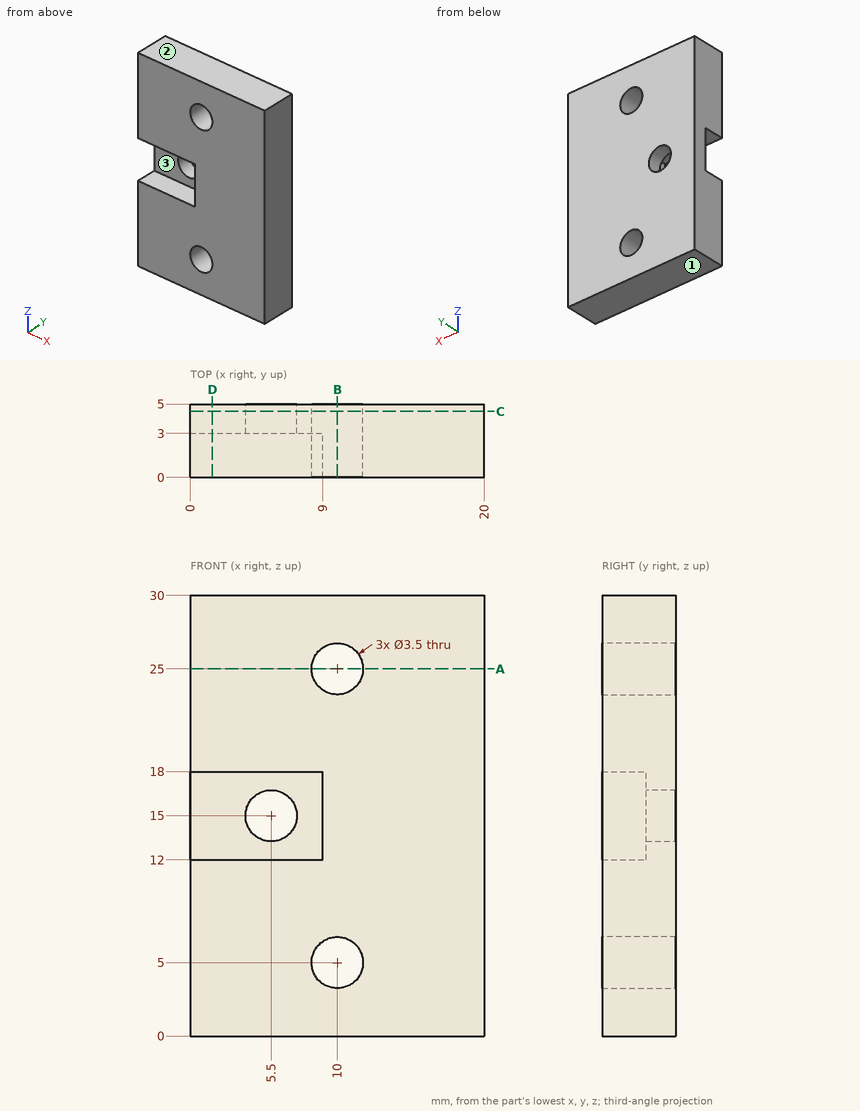
Design review of the part shown in the three views and the two pictorial views. Dimensions are in mm from the part's minimum x, y and z. Round coordinates to 2 decimals unless told otherwise and drop trailing zeros. Order: outer loops, then holes, each group sorted by start corner. A loop starts at its lowest first (then second) coordinate and runs counter-clockwise, first axis right, second up.
(1) Take a section at C-C, the plane y = 4.5. State the section outline as (x, z) points, plus the area to 3 significant figures.
Working result:
outline: (0, 0) - (20, 0) - (20, 30) - (0, 30) - close; hole circle Ø3.5 at (5.5, 15); hole circle Ø3.5 at (10, 5); hole circle Ø3.5 at (10, 25)
area: 571 mm2
(2) For P1, Ø3, axis at x = 6, z = 14.5, coming from the -Y side; P2, Ø0.9, axis at y = 1.5, z = 16.5, coming from the -X side, all flat-tipped, find the tip position at first contact; note any pin that passes through.
Working result:
P1: stops at y = 3
P2: stops at x = 9
(3) Wall thickness on L1, parallel to X at y = 3.9, z = 15; L2, parallel to X at y = 1.9, z = 25; L3, parallel to Z at x = 9.25, y = 1.35: over which ranges is each line inside the solid? List them lowest first.
Working result:
L1: x = 0 to 3.75, 7.25 to 20
L2: x = 0 to 8.25, 11.75 to 20
L3: z = 0 to 3.42, 6.58 to 23.42, 26.58 to 30
(4) Take a section at D-D, the plane x = 1.5. State the section outline as (y, z) points.
Working result:
outline: (0, 0) - (5, 0) - (5, 30) - (0, 30) - (0, 18) - (3, 18) - (3, 12) - (0, 12) - close
(5) Take a section at A-A, the plane z = 25. State the section outline as (x, y) points.
Working result:
outline: (0, 0) - (8.25, 0) - (8.25, 5) - (0, 5) - close; (11.75, 0) - (20, 0) - (20, 5) - (11.75, 5) - close
(6) Take a section at B-B, the plane x = 10. State the section outline as (y, z) points, plus the area to 3 significant figures.
Working result:
outline: (0, 0) - (5, 0) - (5, 3.25) - (0, 3.25) - close; (0, 6.75) - (5, 6.75) - (5, 23.25) - (0, 23.25) - close; (0, 26.75) - (5, 26.75) - (5, 30) - (0, 30) - close
area: 115 mm2
(7) Mouldability with a two-part tool opening along Z and no side actions: class the marked faces 1, 2 and 3 as released by +Z, released by -Z, zero draft, split by the parting line, or undercut.
Working result:
face 1: released by -Z
face 2: released by +Z
face 3: undercut
